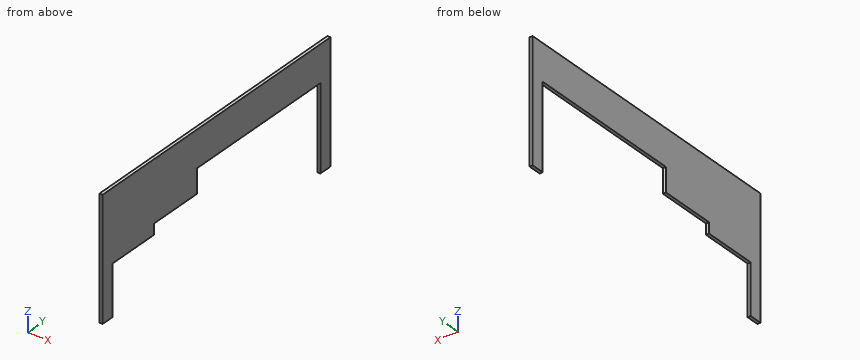
from build123d import *

# Parameters (mm, degrees)
SKETCH_1_W          = 95
SKETCH_1_H          = 38.85
EXTRUDE_1_DEPTH     = 0.5
SKETCH_2_W          = 38.85
SKETCH_2_H          = 95
EXTRUDE_2_DEPTH     = 0.5
CUT_EXTRUDE_1_DEPTH = 110.347085009


with BuildPart() as part:
    # Эскиз1 → Бобышка-Вытянуть1 (new body)
    with BuildSketch(Plane(origin=(0.5, 0, 0), x_dir=(0, -1, 0), z_dir=(-1, 0, 0))):
        with Locations((-53.35, 22.825)):
            Rectangle(SKETCH_1_W, SKETCH_1_H)
    extrude(amount=-EXTRUDE_1_DEPTH)

    # Эскиз2 → Бобышка-Вытянуть2 (add)
    with BuildSketch(Plane.ZY.offset(-0.5)):
        with Locations((22.825, 53.35)):
            Rectangle(SKETCH_2_W, SKETCH_2_H)
    extrude(amount=EXTRUDE_2_DEPTH)

    # Эскиз3 → Вырез-Вытянуть1 (cut, through all)
    with BuildSketch(Plane.ZY):
        Polygon((22.925859733, 27.290305028), (19.520373336, 27.290305028), (19.520373336, 9.916579837), (-2.735278428, 9.916579837), (-2.735278428, 27.290305028), (-2.735278428, 45.262642497), (-2.735278428, 96.642195874), (30.596303396, 96.642195874), (30.596303396, 45.262642497), (22.925859733, 45.262642497), align=None)
    extrude(amount=-CUT_EXTRUDE_1_DEPTH, mode=Mode.SUBTRACT)


solid = part.part
Can you work these out from the model? Positions are in its coordinate system, mm. Give positions to 0.01 mm unless a question says otherwise; leave off trailing zeros. Order: outer loops, then holes, each group sorted by start corner. A loop starts at its lowest first (then second) coordinate and runs counter-clockwise, first axis right, second up. Notation, with made-up numbers: M 52,86 L 84,86 A24 ccw 84,102 Z; hole C -14.5,71.5 d8. An arc over 180 degrees is marked long. One line per question, with ' | ' between items.
Item 1: Suppose I cut it at A-A, the plane z = 25. Write out the boundary of the cut face in (x, y), then the cut area to 3 significant figures.
Answer block:
outline: M 0,5.85 L 1,5.85 L 1,45.26 L 0,45.26 Z; M 0,96.64 L 1,96.64 L 1,100.85 L 0,100.85 Z | area: 43.6 mm2
Item 2: Suppose I cut it at D-D, the plane y = 74. Write out the boundary of the cut face in (x, z).
Answer block:
outline: M 0,30.6 L 1,30.6 L 1,42.25 L 0,42.25 Z
Item 3: Suppose I cut it at B-B, the plane x = 0.15. Write out the boundary of the cut face in (y, z), then the cut area to 3 significant figures.
Answer block:
outline: M 5.85,3.4 L 9.92,3.4 L 9.92,19.52 L 27.29,19.52 L 27.29,22.93 L 45.26,22.93 L 45.26,30.6 L 96.64,30.6 L 96.64,3.4 L 100.85,3.4 L 100.85,42.25 L 5.85,42.25 Z | area: 1,660 mm2
Item 4: Suppose I cut it at C-C, the plane z = 17. Write out the boundary of the cut face in (x, y), then the cut area to 3 significant figures.
Answer block:
outline: M 0,5.85 L 1,5.85 L 1,9.92 L 0,9.92 Z; M 0,96.64 L 1,96.64 L 1,100.85 L 0,100.85 Z | area: 8.27 mm2
Item 5: Please list where these lines run through material, in increasing order: L1, parallel to Y at x = 0.6, z = 30.5; L2, parallel to Y at x = 0.4, z = 10; L3, parallel to Z at x = 0.7, y = 67.5.
Answer block:
L1: y = 5.85 to 45.26, 96.64 to 100.85 | L2: y = 5.85 to 9.92, 96.64 to 100.85 | L3: z = 30.6 to 42.25
Item 6: I'm going to push flat-ended pins straight in: pin 1 Ø0.5 at (x, y) = (0.5, 81.5) entering from -Z; pin 2 Ø0.5 at (x, y) = (0.5, 16) entering from -Z. Where does each tip first touch, or does it pass through?
Answer block:
pin 1: stops at z = 30.6 | pin 2: stops at z = 19.52
